```python
from build123d import *

# Parameters (mm, degrees)
BOSS_EXTRUDE1_DEPTH = 5
SKETCH3_R           = 5
BOSS_EXTRUDE2_DEPTH = 5
BOSS_EXTRUDE3_DEPTH = 2
BOSS_EXTRUDE5_DEPTH = 29
SKETCH6_R           = 2.1
SKETCH6_R_2         = 3
CUT_EXTRUDE1_DEPTH  = 11


with BuildPart() as part:
    # Sketch2 → Boss-Extrude1 (new body)
    with BuildSketch(Plane.XY):
        with BuildLine():
            Line((-35, -12.5), (35, -12.5))
            ThreePointArc((35, -12.5), (43.535533906, -16.035533906), (40, -7.5))
            ThreePointArc((40, -7.5), (0, 0), (-40, -7.5))
            ThreePointArc((-40, -7.5), (-43.535533906, -16.035533906), (-35, -12.5))
        make_face()
    extrude(amount=BOSS_EXTRUDE1_DEPTH)

    # Sketch3 → Boss-Extrude2 (add)
    with BuildSketch(Plane.XY.offset(5)):
        with Locations((-40, -12.5)):
            Circle(SKETCH3_R)
        with Locations(Location((40, -12.5, 0), (0, 0, 180))):  # turned: the seam where the file's is
            Circle(SKETCH3_R)
    extrude(amount=BOSS_EXTRUDE2_DEPTH)

    # Sketch4 → Boss-Extrude3 (add)
    with BuildSketch(Plane(origin=(0, 0, 0), x_dir=(-1, 0, 0), z_dir=(0, 0, -1))):
        with BuildLine():
            Line((-40, 17.5), (-70, 17.5))
            Line((-70, 17.5), (-70, 15.5))
            Line((-70, 15.5), (-43.655276341, -9.088408748))
            ThreePointArc((-43.655276341, -9.088408748), (-41.992742299, -7.914263622), (-40, -7.5))
            ThreePointArc((-40, -7.5), (-26.428535361, -3.209517668), (-12.417905405, -0.700506038))
            ThreePointArc((-12.417905405, -0.700506038), (-23.477058659, 12.539816482), (-40, 17.5))
        make_face()
        with BuildLine():
            ThreePointArc((61.213203436, 8.713203436), (34.317115595, 16.95682985), (12.417905405, -0.700506038))
            ThreePointArc((12.417905405, -0.700506038), (26.428535361, -3.209517668), (40, -7.5))
            ThreePointArc((40, -7.5), (41.913417162, -7.880602337), (43.535533906, -8.964466094))
            Line((43.535533906, -8.964466094), (61.213203436, 8.713203436))
        make_face()
    extrude(amount=-BOSS_EXTRUDE3_DEPTH)

    # Sketch5 → Boss-Extrude5 (add)
    with BuildSketch(Plane.XY.offset(2)):
        with BuildLine():
            Line((-59.798989873, 7.298989873), (-61.213203436, 8.713203436))
            ThreePointArc((-61.213203436, 8.713203436), (-33.506811582, 16.788880214), (-11.809221376, -2.2393957))
            Line((-11.809221376, -2.2393957), (-13.688606618, -2.923435987))
            ThreePointArc((-13.688606618, -2.923435987), (-33.93969081, 14.836288199), (-59.798989873, 7.298989873))
        make_face()
        with BuildLine():
            Line((40, 17.5), (70, 17.5))
            Line((70, 17.5), (70, 15.5))
            Line((70, 15.5), (40, 15.5))
            ThreePointArc((40, 15.5), (23.939859782, 10.43625724), (13.688606618, -2.923435987))
            Line((13.688606618, -2.923435987), (11.809221376, -2.2393957))
            ThreePointArc((11.809221376, -2.2393957), (22.792706909, 12.074561329), (40, 17.5))
        make_face()
    extrude(amount=BOSS_EXTRUDE5_DEPTH)

    # Sketch6 → Cut-Extrude1 (cut, through all)
    with BuildSketch(Plane.XY.offset(10)):
        with Locations((-40, -12.5)):
            Circle(SKETCH6_R)
        with Locations((40, -12.5)):
            Circle(SKETCH6_R)
        with Locations((0, -4)):
            Circle(SKETCH6_R_2)
        with Locations((-6.5, -8.5)):
            Circle(SKETCH6_R_2)
        with Locations((6.5, -8.5)):
            Circle(SKETCH6_R_2)
    extrude(amount=-CUT_EXTRUDE1_DEPTH, mode=Mode.SUBTRACT)


solid = part.part
```
Part model, mm, in its own coordinate system. A direction names the side the tool comes from. Give positions to 0.01 mm unless a question says otherwise; leave off trailing zeros. Loops run counter-clockwise (first coordinate to the right, second up) from the corner with the lowest first, then second, coordinate; pieces in that order, holes last. Notation, with made-up numbers: M 70.5,67 L 104.5,67 A26 cw 104.5,88 Z; hole C 16.25,-16 d5. An arc over 180 degrees is marked long. Return JSON: item names as keys, results as strings.
1) Saw through at A-A, the plane x = 0. List the corners of the cut face in (y, z).
Calculated:
{"outline": "M -12.5,0 L -7,0 L -7,5 L -12.5,5 Z; M -1,0 L 0,0 L 0,5 L -1,5 Z"}
2) Drill centre lines: line 1 (Y direction, x = 40, z = 6); line 2 (X direction, y = 13, z = 25); line 3 (Y direction, x = 0, z = 3.7). Where is each one in solid material? Low to high.
Calculated:
{"line 1": "y = -17.5 to -14.6, -10.4 to -7.5, 15.5 to 17.5", "line 2": "x = -55.8 to -51.57, -28.43 to -24.2, 24.2 to 28.43", "line 3": "y = -12.5 to -7, -1 to 0"}
3) Saw through at B-B, the plane z = 8. List the corners of the cut face in (x, y).
Calculated:
{"outline": "M -61.21,8.71 L -59.8,7.3 A28 cw -13.69,-2.92 L -11.81,-2.24 A30 ccw Z; C -40,-12.5 d10; M 11.81,-2.24 L 13.69,-2.92 A28 cw 40,15.5 L 70,15.5 L 70,17.5 L 40,17.5 A30 ccw Z; C 40,-12.5 d10; hole C -40,-12.5 d4.2; hole C 40,-12.5 d4.2"}
4) Saw through at C-C, the plane z = 24.5. List the corners of the cut face in (x, y).
Calculated:
{"outline": "M -61.21,8.71 L -59.8,7.3 A28 cw -13.69,-2.92 L -11.81,-2.24 A30 ccw Z; M 11.81,-2.24 L 13.69,-2.92 A28 cw 40,15.5 L 70,15.5 L 70,17.5 L 40,17.5 A30 ccw Z"}
5) Pull direction X, two halves, no side cores. Call faces 1 (the face through (40, -10, 10)), 2 (the face through (0, -12.5, 2)), 3 (the face through (-27.262, -3.418, 3.479)): released by +X, released by -X, zero draft, split by the parting line, or undercut.
Calculated:
{"face 1": "zero draft", "face 2": "undercut", "face 3": "released by -X"}
6) 3-axis set-ups, long thin cutter, end or side, ignore diameter. For faces 4 (the face through (-40, -15, 10)), 5 (the face through (55, 17.5, 15)), 6 (the face through (27.62, -3.51, 3.48)), 7 (the face through (-37, 3, 2)), 8 (the face through (-3.64, -7.6, 2.54)): which of +Z, -Z, +X, -X, +Y, -Y reach the whole face in a straight line?
Calculated:
{"face 4": "+Z, +X, -X, -Y", "face 5": "+Z, -Z, +X, -X, +Y", "face 6": "+Z, +X", "face 7": "+Z", "face 8": "+Z, -Z"}
7) Saw through at D-D, the plane x = 17. List the corners of the cut face in (y, z), then the cut area to 3 significant figures.
Calculated:
{"outline": "M -12.5,0 L 6.76,0 L 6.76,31 L 3.47,31 L 3.47,2 L -1.32,2 L -1.32,5 L -12.5,5 Z", "area": "168 mm2"}
8) Flat gauge pins, fed straight in: pin 1 Ø4 at (x, z) = (32.5, 3.5) entering from -Y; pin 2 Ø19.5 at (x, y) = (-46, 3) entering from +Z; pin 3 Ø6.5 at (x, y) = (-40, -12.5) entering from +Z; pin 4 Ø6 at (x, y) = (40, 4) entering from -Z. Where does each tip first touch, or does it go through?
Calculated:
{"pin 1": "stops at y = -12.5", "pin 2": "stops at z = 2", "pin 3": "stops at z = 10", "pin 4": "stops at z = 0"}
